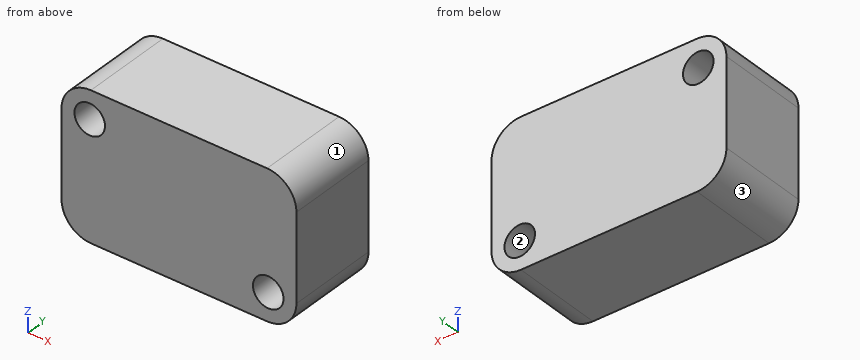
Autodesk Inventor part; units mm, degrees
ref_plane "YZ Plane" through (0, 0, 0) normal (1, 0, 0) x (0, 1, 0)
ref_plane "XZ Plane" through (0, 0, 0) normal (0, 1, 0) x (-1, 0, 0)
ref_plane "XY Plane" through (0, 0, 0) normal (0, 0, 1) x (1, 0, 0)
sketch "Sketch1" plane through (0, 0, 0) normal (0, 1, 0) x (-1, 0, 0)
  line L0 (0, 0) -> (25.4, 0)
  line L1 (25.4, 0) -> (25.4, -15.748)
  line L2 (25.4, -15.748) -> (0, -15.748)
  line L3 (0, -15.748) -> (0, 0)
  dimension "d0" = 25.4
  dimension "d1" = 15.748
extrude "Extrusion1" add sketch "Sketch1" along normal blind 9.906
sketch "Sketch2" plane through (0, 9.906, 0) normal (0, 1, 0) x (1, 0, 0)
  line L0 (-25.4, 0) -> (0, 0)
  line L1 (0, 0) -> (0, 15.748)
  line L2 (0, 15.748) -> (-25.4, 15.748)
  line L3 (-25.4, 15.748) -> (-25.4, 0)
  point P0 (-3.048, 12.7)
  point P1 (-22.352, 3.048)
  dimension "d5" = 3.048
  dimension "d6" = 3.048
  dimension "d7" = 3.048
  dimension "d8" = 3.048
hole "Hole1" at (-3.048, 9.906, -12.7) at (-22.352, 9.906, -3.048) direction (0, -1, 0) diameter 3.302 end through all
fillet "Fillet1" radius 3.175 4 edges at (-25.4, 4.953, 0) (-25.4, 4.953, -15.748) (0, 4.953, -15.748) (0, 4.953, 0)
ref_plane "Work Plane1" through (0, 4.953, 0) normal (0, 1, 0) x (1, 0, 0)
properties part number "LimitSwitch"
Input: part model. Units: mm. Frame: model coordinates. Face numbers are marked on the shaded views. Round coordinates to 2 decimals unless told otherwise and drop trailing zeros. Loops run counter-clockwise (first coordinate to the right, second up) from the corner with the lowest first, then second, coordinate; pieces in that order, holes last. Notation, with made-up numbers: (-17.5, -17.5) -> (12.5, -17.5) arc R24 ccw to (12.5, 12.5) -> close; hole circle Ø9 at (-36, 37.25). An arc over 180 degrees is marked (long way). Answer as a JSON object with one key per item and string values. Group by question number.
1) Section query C-C on z = -0.75. Output: boundary loops of the cut face in (x, y).
2) Ray query, L1, parallel to X at y = 3.5, z = -12.7; L2, parallel to X at y = 3, z = -2.75; L3, parallel to Z at x = -3.75, y = 4.75. Return the intervals inside material, ascending.
3) Section query A-A on z = -14. Output: boundary loops of the cut face in (x, y), plus the area to 3 significant figures.
4) Draft query along X for the marked faces 1, 2 and 3. Return one class per face: +X half, -X half, draft (parallel to the pull), parting line (faces both ways), or undercut.
5) Pin query (flat end, axial travel): pin 1 (4 mm diameter, centred on x = -11.5, z = -4, fed in from -Y); pin 2 (2.5 mm diameter, centred on x = -22.352, z = -3.048, fed in from +Y); pin 3 (2 mm diameter, centred on y = 1.5, z = -2, fed in from -X). Return the tip coordinate at first contact, or that it passes through.
6) Section query B-B on y = 5.5. Output: boundary loops of the cut face in (x, z) (3 decimals).
Reply:
{
 "1": {"outline": "(-24.27, 0) -> (-1.13, 0) -> (-1.13, 9.91) -> (-24.27, 9.91) -> close"},
 "2": {"L1": "x = -25.4 to -4.7, -1.4 to 0", "L2": "x = -25.37 to -23.98, -20.73 to -0.03", "L3": "z = -15.75 to -14.19, -11.21 to 0"},
 "3": {"outline": "(-25.06, 0) -> (-4.07, 0) -> (-4.07, 9.91) -> (-25.06, 9.91) -> close; (-2.03, 0) -> (-0.34, 0) -> (-0.34, 9.91) -> (-2.03, 9.91) -> close", "area": "225 mm2"},
 "4": {"face 1": "+X half", "face 2": "undercut", "face 3": "-X half"},
 "5": {"pin 1": "stops at y = 0", "pin 2": "passes through", "pin 3": "stops at x = -25.4"},
 "6": {"outline": "(-25.4, -12.573) arc R3.175 ccw to (-22.225, -15.748) -> (-3.175, -15.748) arc R3.175 ccw to (0, -12.573) -> (0, -3.175) arc R3.175 ccw to (-3.175, 0) -> (-22.225, 0) arc R3.175 ccw to (-25.4, -3.175) -> close; hole circle Ø3.302 at (-22.352, -3.048); hole circle Ø3.302 at (-3.048, -12.7)"}
}
